from build123d import *

# Parameters (mm, degrees)
EXTRUDE_1_DEPTH = 5


with BuildPart() as part:
    # Эскиз1 → Повернуть1 (revolve)
    with BuildSketch(Plane(origin=(0, 0, 0), x_dir=(0, 0, -1), z_dir=(1, 0, 0))):
        Polygon((0, 0), (0, 39), (-4, 39), (-4, 35), (-34, 5), (-34, 0), align=None)
    revolve(axis=Axis((0, 0, 926.802095793), (0, 0, -1)))

    # Эскиз2 → Бобышка-Вытянуть1 (add)
    with BuildSketch(Plane(origin=(0, 0, 0), x_dir=(-1, 0, 0), z_dir=(0, 0, -1))):
        Polygon((12.5, -15.5), (-12.5, -15.5), (-15.5, -12.5), (-15.5, 12.5), (-12.5, 15.5), (12.5, 15.5), (15.5, 12.5), (15.5, -12.5), align=None)
    extrude(amount=EXTRUDE_1_DEPTH)


solid = part.part
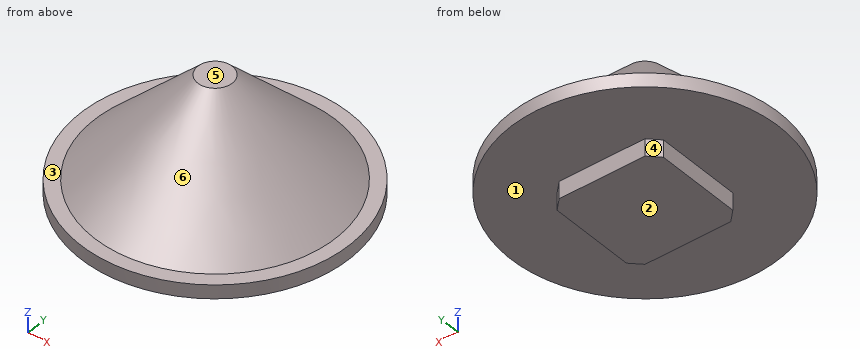
The listing builds one solid part. Answer for the finished solid, in the listing's coordinates (mm). Face numbers are marked on the shaded views. A direction names the side the tool comes from. Coordinates: 2 decimals unless noted, no trailing zeros. Order: outer loops, then holes, each group sorted by start corner. A loop starts at its lowest first (then second) coordinate and runs counter-clockwise, first axis right, second up.
Q1. Consider line 1 (Z direction, x = -21.5, y = -32.5); line 2 (X direction, y = 6, z = -3); line 3 (X direction, y = -25.5, z = 9). Determine where each line is inside the solid, lowest interval first.
Q2. Which of the six approach directions +Z, -Z, +X, -X, +Y, -Y give full straight-line access (tool end or side, diameter ignored) to the marked faces 1, 2 and 3?
Q3. Given P1, Ø1.5, axis at y = 3.5, z = -3.5, coming from the -X side; P2, Ø10, axis at y = -9.5, z = 6, coming from the +X side; P3, Ø1, axis at y = 0, z = 7, coming from the +X side, each flat-ended and moving along its own axis, determine where each tip first touches the part or whether it passes through.
Q4. A cutting plane is placed at A-A, the plane x = 0. Write down the section's boundary in (y, z).
Q5. A cutting plane is placed at D-D, the plane z = 28.5. Write down the section's boundary in (x, y).
Q6. A cutting plane is placed at C-C, the plane z = 17.5. Write down the section's boundary in (x, y).
Q7. For a pull along X with two mould halves and no side action, classify the marked faces 4, 5 and 6 as pulls with the +X half, pulls with the -X half, needs draft (parallel to the pull), parting line crosses it, or undercut.
Answers follow:
1. line 1: z = 0 to 4
1. line 2: x = -15.5 to 15.5
1. line 3: x = -15.8 to 15.8
2. face 1: -Z
2. face 2: -Z, +X, -X, +Y, -Y
2. face 3: +Z
3. P1: stops at x = -15.5
3. P2: stops at x = 38.69
3. P3: stops at x = 32.5
4. outline: (-39, 0) - (-15.5, 0) - (-15.5, -5) - (15.5, -5) - (15.5, 0) - (39, 0) - (39, 4) - (35, 4) - (5, 34) - (-5, 34) - (-35, 4) - (-39, 4) - close
5. outline: circle Ø21 at (0, 0)
6. outline: circle Ø43 at (0, 0)
7. face 4: pulls with the -X half
7. face 5: needs draft
7. face 6: parting line crosses it
